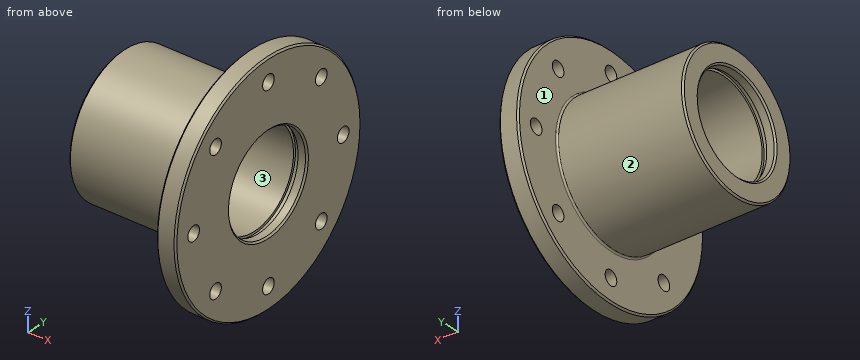
```python
from build123d import *

# Parameters (mm, degrees)
M4_GEWINDEBOHRUNG1_D            = 3.3
M4_GEWINDEBOHRUNG1_DEPTH        = 13
M4_GEWINDEBOHRUNG1_TIP          = 0.991420021
SKIZZE8_R                       = 2.25
SCHNITT_LINEAR_AUSTRAGEN1_DEPTH = 68.948509917


with BuildPart() as part:
    # Skizze2 → Rotation1 (revolve)
    with BuildSketch(Plane(origin=(0, 0, 0), x_dir=(1, 0, 0), z_dir=(0, 1, 0)), mode=Mode.PRIVATE) as rotation1_sk:
        with BuildLine():
            Line((33.5, 21.002136322), (33.5, 15))
            Line((33.5, 15), (40.8, 15))
            Line((40.8, 15), (40.8, 15.75))
            Line((40.8, 15.75), (42.2, 15.75))
            Line((42.2, 15.75), (42.2, 15))
            Line((42.2, 15), (44.5, 15))
            Line((44.5, 15), (45, 15.5))
            Line((45, 15.5), (45, 20))
            Line((45, 20), (45, 35.5))
            Line((45, 35.5), (44.5, 36))
            Line((44.5, 36), (39.5, 36))
            Line((39.5, 36), (39, 35.5))
            Line((39, 35.5), (39, 21.502136322))
            ThreePointArc((39, 21.502136322), (38.853553391, 21.148582931), (38.5, 21.002136322))
            Line((38.5, 21.002136322), (33.5, 21.002136322))
        make_face()
        Polygon((0, 20.502136322), (0, 15.5), (0.5, 15), (2.8, 15), (2.8, 15.75), (4.2, 15.75), (4.2, 15), (33.5, 15), (33.5, 21.002136322), (0.5, 21.002136322), align=None)
    revolve(rotation1_sk.sketch.rotate(Axis((0, 0, 0), (1, 0, 0)), 180), axis=Axis((0, 0, 0), (1, 0, 0)))

    # M4 Gewindebohrung1
    with Locations(Plane(origin=(67, 14.142135624, 14.142135624), x_dir=(0, 0, 1), z_dir=(1, 0, 0))):
        with Locations((0, 0), (-14.142135624, -5.857864376), (-28.284271248, 0), (-34.142135624, 14.142135624), (-28.284271248, 28.284271248), (-14.142135624, 34.142135624), (0, 28.284271248), (5.857864376, 14.142135624)):
            Hole(M4_GEWINDEBOHRUNG1_D / 2, depth=M4_GEWINDEBOHRUNG1_DEPTH)
            with Locations((0, 0, -(M4_GEWINDEBOHRUNG1_DEPTH + M4_GEWINDEBOHRUNG1_TIP / 2))):  # 118° drill point
                Cone(0, M4_GEWINDEBOHRUNG1_D / 2, M4_GEWINDEBOHRUNG1_TIP, mode=Mode.SUBTRACT)

    # Skizze8 → Schnitt-Linear austragen1 (cut, through all)
    with BuildSketch(Plane(origin=(45, 0, 0), x_dir=(0, 0, -1), z_dir=(1, 0, 0))):
        with Locations((0, 29)):
            Circle(SKIZZE8_R)
        with Locations((20.506096654, 20.506096654)):
            Circle(SKIZZE8_R)
        with Locations((29, 0)):
            Circle(SKIZZE8_R)
        with Locations((20.506096654, -20.506096654)):
            Circle(SKIZZE8_R)
        with Locations((0, -29)):
            Circle(SKIZZE8_R)
        with Locations((-20.506096654, -20.506096654)):
            Circle(SKIZZE8_R)
        with Locations((-29, 0)):
            Circle(SKIZZE8_R)
        with Locations((-20.506096654, 20.506096654)):
            Circle(SKIZZE8_R)
    extrude(amount=-SCHNITT_LINEAR_AUSTRAGEN1_DEPTH, mode=Mode.SUBTRACT)


solid = part.part
```
Source: CAD feature listing. Evaluate the final solid. Frame: model axes, mm. Face numbers are marked on the shaded views. Give positions to 0.01 mm unless a question says otherwise; leave off trailing zeros. Write each loop counter-clockwise with the first axis right and the second up, starting at its lowest first coordinate (ties: lowest second). Pieces come first, ordered by that corner, then holes. Notation, with made-up numbers: (16, -1) - (61, -1) arc R18 cw to (61, 6) - close; hole circle Ø2 at (11, 58.25). An arc over 180 degrees is marked (long way). One line per item, written item: value. Start each with the question number.
Q1. Material intervals for probe 1 along Y at (x, z) = (41.1, 0); probe 2 along Y at (x, z) = (43.45, 0); probe 3 along X at (y, z) = (-29.5, 11), sorted ascending. Write a range as from..to.
Q2. Draft query along Y for the marked faces 1, 2 and 3. Return one class per face: +Y half, -Y half, draft (parallel to the pull), parting line (faces both ways), or undercut.
Q3. First-contact query: pin 1 Ø10 at (x, z) = (14, -28.5) entering from +Y; pin 2 Ø10 at (x, y) = (26.5, 15) entering from +Z; pin 3 Ø1.5 at (x, z) = (12, -7) entering from -Y; pin 4 Ø5 at (x, y) = (18, -12.5) entering from -Z. Flat tips, straight axial feed; report the tip coordinate or a pass-through.
Q4. Section query B-B, the plane y = 0. Count the separate pieces of the cut face and the enclosed holes in it, then the cut area to 3 significant figures.
Q5. Section query A-A, the plane x = 34. Return the cut outline in (y, z).
Answer:
1. probe 1: y = -36..-31.25, -26.75..-15.75, 15.75..26.75, 31.25..36
1. probe 2: y = -36..-31.25, -26.75..-15, 15..26.75, 31.25..36
1. probe 3: x = 39..45
2. face 1: draft
2. face 2: parting line
2. face 3: undercut
3. pin 1: passes through
3. pin 2: stops at z = 18.47
3. pin 3: stops at y = -20.05
3. pin 4: stops at z = -18.47
4. separate pieces: 4
4. enclosed holes: 0
4. area: 661 mm2
5. outline: circle Ø42 at (0, 0); hole circle Ø30 at (0, 0)
